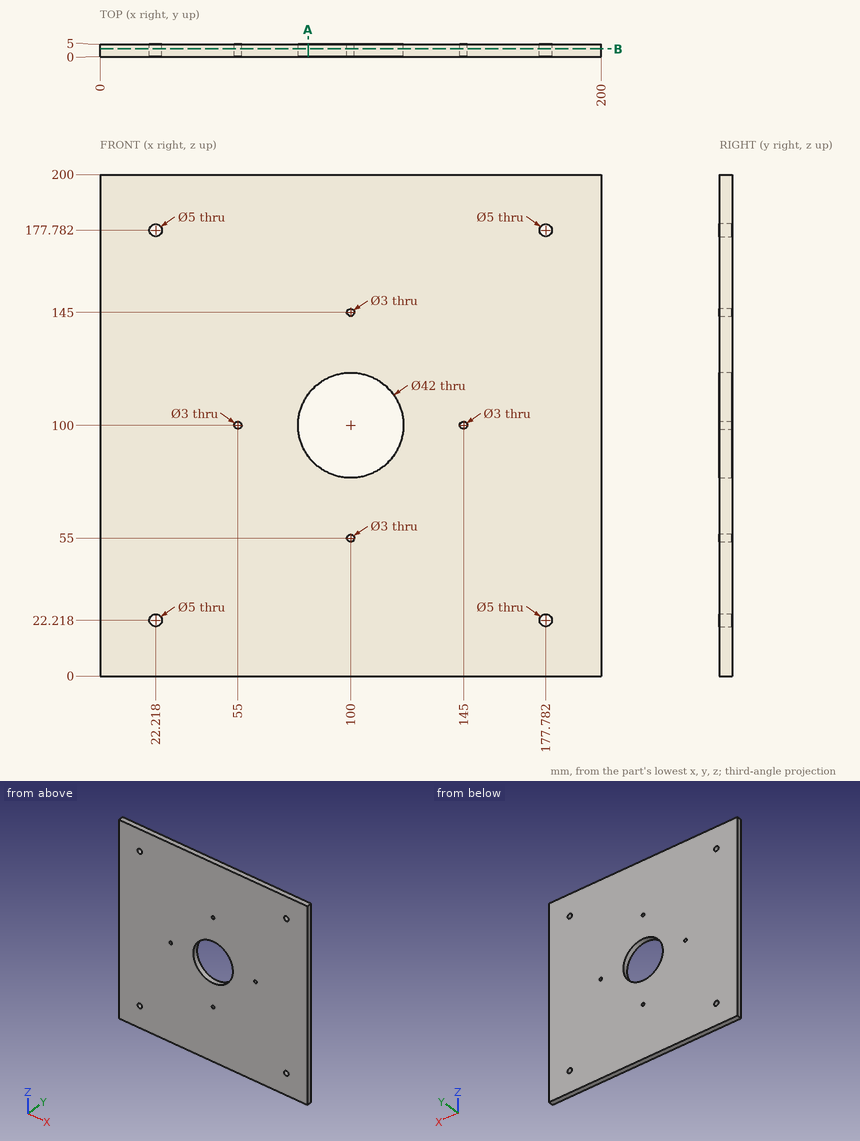
Design review of the part shown in the three views and the two pictorial views. Dimensions are in mm from the part's minimum x, y and z. Coordinates: 2 decimals unless noted, no trailing zeros. Order: outer loops, then holes, each group sorted by start corner. A loop starts at its lowest first (then second) coordinate and runs counter-clockwise, first axis right, second up.
Item 1: For line 1 (X direction, y = 3.75, z = 100); line 2 (Z direction, x = 55, y = 1.6); line 3 (Z direction, x = 175.5, y = 1.65) (1 decimal), list the stretches that pass through material, from the lowest coordinate up.
Item 2: Take a section at B-B, the plane y = 3.05. Count the separate pieces of the cut face and the enclosed holes in it, then the cut area to 3 significant figures.
Item 3: Take a section at A-A, the plane x = 83. Write out the cut boundary in (y, z), then the cut area to 3 significant figures.
Item 4: For pin 1 Ø25 at (x, z) = (100, 100) entering from +Y, flat-tipped, find the tip position at first contact; note if it passes through.
The answers:
1. line 1: x = 0 to 53.5, 56.5 to 79, 121 to 143.5, 146.5 to 200
1. line 2: z = 0 to 98.5, 101.5 to 200
1. line 3: z = 0 to 21.2, 23.2 to 176.8, 178.8 to 200
2. separate pieces: 1
2. enclosed holes: 9
2. area: 38,500 mm2
3. outline: (0, 0) - (5, 0) - (5, 87.67) - (0, 87.67) - close; (0, 112.33) - (5, 112.33) - (5, 200) - (0, 200) - close
3. area: 877 mm2
4. pin 1: passes through
